Source: CAD feature listing. Evaluate the final solid. Frame: model axes, mm. Face numbers are marked on the shaded views. Give positions to 0.01 mm unless a question says otherwise; leave off trailing zeros. Order: outer loops, then holes, each group sorted by start corner. A loop starts at its lowest first (then second) coordinate and runs counter-clockwise, first axis right, second up. Notation, with made-up numbers: (-25, 67) - (28, 67) arc R20 cw to (28, 94) - close; hole circle Ø4 at (-12.5, -23.5). An arc over 180 degrees is marked (long way). One line per item, written item: value. Start each with the question number.
from build123d import *

# Parameters (mm, degrees)
SKETCH2_R               = 15
BOSS_EXTRUDE1_DEPTH     = 32.5
CUT_EXTRUDE1_DEPTH      = 50
CUT_EXTRUDE1_DEPTH_BACK = 50
SKETCH3_R               = 13
SKETCH5_R               = 20
BOSS_EXTRUDE2_DEPTH     = 5
FILLET1_R               = 2


with BuildPart() as part:
    # Sketch2 → Boss-Extrude1 (new body)
    with BuildSketch(Plane(origin=(0, 0, 0), x_dir=(1, 0, 0), z_dir=(0, 1, 0))):
        with Locations(Location((0, 0, 0), (0, 0, 270))):
            Circle(SKETCH2_R)
    extrude(amount=BOSS_EXTRUDE1_DEPTH)

    # Sketch3 → Cut-Extrude1 (cut, two sides: drawn at the far end of the back side and taken through both)
    with BuildSketch(Plane.XY.offset(-CUT_EXTRUDE1_DEPTH_BACK)):
        Circle(SKETCH3_R)
    extrude(amount=CUT_EXTRUDE1_DEPTH + CUT_EXTRUDE1_DEPTH_BACK, mode=Mode.SUBTRACT)

    # Sketch5 → Boss-Extrude2 (add)
    with BuildSketch(Plane(origin=(0, 32.5, 0), x_dir=(1, 0, 0), z_dir=(0, 1, 0))):
        with Locations(Location((0, 0, 0), (0, 0, 270))):
            Circle(SKETCH5_R)
    extrude(amount=BOSS_EXTRUDE2_DEPTH)

    # Fillet1
    fillet1_edges = [part.edges().sort_by_distance(p)[0] for p in [
        (0, 32.5, -20),
        (0, 32.5, -15),
    ]]
    fillet(fillet1_edges, radius=FILLET1_R)


solid = part.part
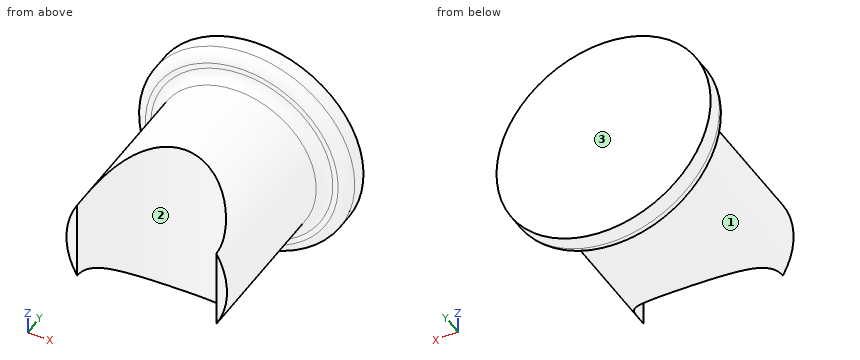
1. Section C-C on y = 27. Return the cut outline in (x, z).
2. Ray query, L1, parallel to Z at x = 0.5, y = 26; L2, parallel to Y at x = -12.5, z = 11.5; L3, parallel to X at y = 16, z = 9. Return the intervals inside material, ascending.
3. Section B-B on x = 0. Return the cut outline in (y, z).
4. Contact query for flat-ended pins moving along their axis: pin 1 Ø5 at (x, z) = (1, -11) entering from -Y; pin 2 Ø8 at (y, z) = (33.5, 12) entering from -X; pin 3 Ø3 at (y, z) = (12.5, 5.5) entering from -X. Output: stop coordinate, or through.
5. Draft query along X for the marked faces 1, 2 and 3. Return one class per face: pulls with the +X half, pulls with the -X half, needs draft (parallel to the pull), parting line crosses it, or undercut.
6. Section A-A on z = 0. Return the cut outline in (x, y).
Data:
1. outline: circle Ø30 at (0, 0)
2. L1: z = -14.99 to 14.99
2. L2: y = 32.5 to 37.5
2. L3: x = -12 to 12
3. outline: (13, -15) - (30.5, -15) arc R2 cw to (32.5, -17) - (32.5, -18) arc R2 ccw to (34.5, -20) - (37.5, -20) - (37.5, 20) - (34.5, 20) arc R2 ccw to (32.5, 18) - (32.5, 17) arc R2 cw to (30.5, 15) - (13, 15) - close
4. pin 1: stops at y = 12.52
4. pin 2: stops at x = -18.28
4. pin 3: stops at x = -14.46
5. face 1: parting line crosses it
5. face 2: undercut
5. face 3: needs draft
6. outline: (-20, 34.5) arc R2 ccw to (-18, 32.5) - (-17, 32.5) arc R2 cw to (-15, 30.5) - (-15, 0) - (-13, 0) arc R13 cw to (13, 0) - (15, 0) - (15, 30.5) arc R2 cw to (17, 32.5) - (18, 32.5) arc R2 ccw to (20, 34.5) - (20, 37.5) - (-20, 37.5) - close
